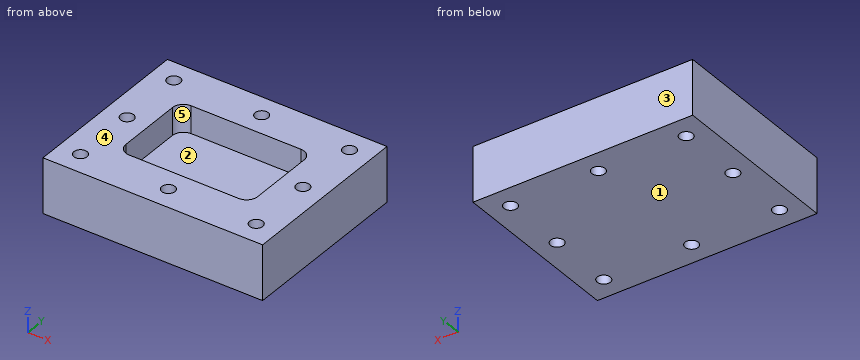
from build123d import *

# Parameters (mm, degrees)
SKETCH1_W          = 200
SKETCH1_H          = 160
BASE_EXTRUDE_DEPTH = 50
CUT_EXTRUDE1_DEPTH = 25
SKETCH3_R          = 6
CUT_EXTRUDE2_DEPTH = 138.477270849


with BuildPart() as part:
    # Sketch1 → Base-Extrude (new body)
    with BuildSketch(Plane.XY):
        Rectangle(SKETCH1_W, SKETCH1_H)
    extrude(amount=-BASE_EXTRUDE_DEPTH)

    # Sketch2 → Cut-Extrude1 (cut)
    with BuildSketch(Plane.XY):
        with BuildLine():
            Line((-50, 40), (50, 40))
            ThreePointArc((50, 40), (57.071067812, 37.071067812), (60, 30))
            Line((60, 30), (60, -30))
            ThreePointArc((60, -30), (57.071067812, -37.071067812), (50, -40))
            Line((50, -40), (-50, -40))
            ThreePointArc((-50, -40), (-57.071067812, -37.071067812), (-60, -30))
            Line((-60, -30), (-60, 30))
            ThreePointArc((-60, 30), (-57.071067812, 37.071067812), (-50, 40))
        make_face()
    extrude(amount=-CUT_EXTRUDE1_DEPTH, mode=Mode.SUBTRACT)

    # Sketch3 → Cut-Extrude2 (cut, through all)
    with BuildSketch(Plane.XY):
        with Locations((-80, 60)):
            Circle(SKETCH3_R)
        with Locations((-80, 0)):
            Circle(SKETCH3_R)
        with Locations((-80, -60)):
            Circle(SKETCH3_R)
        with Locations((80, -60)):
            Circle(SKETCH3_R)
        with Locations((80, 0)):
            Circle(SKETCH3_R)
        with Locations((80, 60)):
            Circle(SKETCH3_R)
        with Locations((0, -60)):
            Circle(SKETCH3_R)
        with Locations((0, 60)):
            Circle(SKETCH3_R)
    extrude(amount=-CUT_EXTRUDE2_DEPTH, mode=Mode.SUBTRACT)


solid = part.part
Could you check a few things on this model? Use its own coordinates, in mm. Face numbers are marked on the shaded views. A direction names the side the tool comes from. Give positions to 0.01 mm unless a question says otherwise; leave off trailing zeros. Loops run counter-clockwise (first coordinate to the right, second up) from the corner with the lowest first, then second, coordinate; pieces in that order, holes last. Notation, with made-up numbers: (26, -17) -> (77, -17) arc R5 cw to (77, -8) -> close; hole circle Ø1 at (81.5, -6). An arc over 180 degrees is marked (long way). Answer as CSV lines item,"result". Start each with the question number.
(1) If we section it at B-B on y = 0: Write out the boundary of the cut face in (x, z).
(2) If we section it at C-C on z = -39.5: Count the separate pieces of the cut face and the enclosed holes in it, then the cut area to 3 significant figures.
(3) If we section it at D-D on x = -80: Write out the boundary of the cut face in (y, z).
(4) I need wall thicknesses on probe 1 along Y at (x, z) = (0, -14); probe 2 along Y at (x, z) = (0, -27); probe 3 along Y at (x, z) = (-80, -34). Which ranges of each line are inside material? Lowest first, please.
(5) If we section it at A-A on x = 0: Write out the boundary of the cut face in (y, z).
(6) I'm going to push a flat-ended pin straight in: pin 1 Ø2 at (x, y) = (36.5, -33) entering from +Z. Where does the tip first touch, or does it pass through?
(7) We'd pull the mould along Y, two halves only. Please class the marked faces 1, 2 and 3: released by +Y, released by -Y, zero draft, split by the parting line, or undercut.
(8) Which directions (+Z, -Z, +X, -X, +Y, -Y) give clear straight access to the entire face, cutting with the end or side of a thin tool? Please do the marked faces 4 and 5.
Computed:
1,outline,"(-100, -50) -> (-86, -50) -> (-86, 0) -> (-100, 0) -> close; (-74, -50) -> (74, -50) -> (74, 0) -> (60, 0) -> (60, -25) -> (-60, -25) -> (-60, 0) -> (-74, 0) -> close; (86, -50) -> (100, -50) -> (100, 0) -> (86, 0) -> close"
2,separate pieces,"1"
2,enclosed holes,"8"
2,area,"31,100 mm2"
3,outline,"(-80, -50) -> (-66, -50) -> (-66, 0) -> (-80, 0) -> close; (-54, -50) -> (-6, -50) -> (-6, 0) -> (-54, 0) -> close; (6, -50) -> (54, -50) -> (54, 0) -> (6, 0) -> close; (66, -50) -> (80, -50) -> (80, 0) -> (66, 0) -> close"
4,probe 1,"y = -80 to -66, -54 to -40, 40 to 54, 66 to 80"
4,probe 2,"y = -80 to -66, -54 to 54, 66 to 80"
4,probe 3,"y = -80 to -66, -54 to -6, 6 to 54, 66 to 80"
5,outline,"(-80, -50) -> (-66, -50) -> (-66, 0) -> (-80, 0) -> close; (-54, -50) -> (54, -50) -> (54, 0) -> (40, 0) -> (40, -25) -> (-40, -25) -> (-40, 0) -> (-54, 0) -> close; (66, -50) -> (80, -50) -> (80, 0) -> (66, 0) -> close"
6,pin 1,"stops at z = -25"
7,face 1,"zero draft"
7,face 2,"undercut"
7,face 3,"released by +Y"
8,face 4,"+Z, +X, -X, +Y, -Y"
8,face 5,"+Z"
